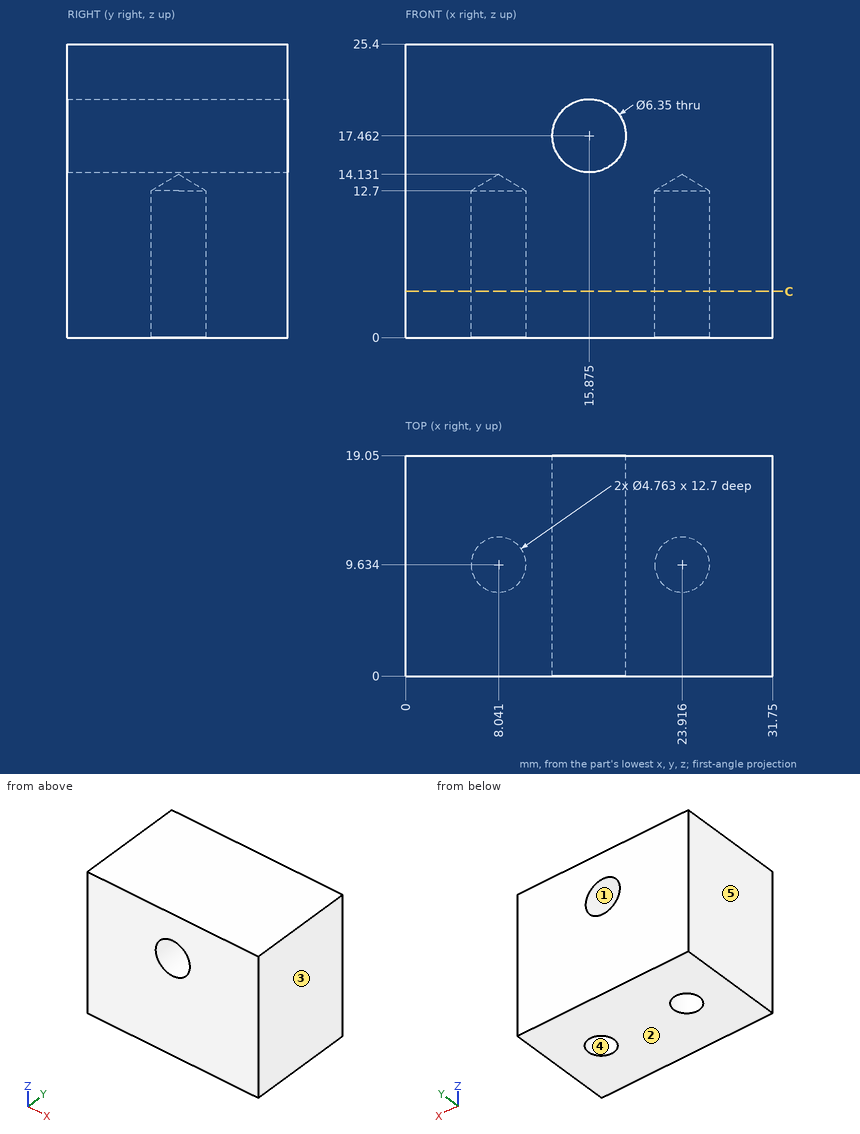
Print and shaded views of the part. All mm, measured from the part's lowest x, y and z. A direction names the side the tool comes from. Round coordinates to 2 decimals unless told otherwise and drop trailing zeros. One line per question, with ' | ' between items.
1. Band-saw the part on C-C, the plane z = 4. Give the number of separate pieces and of enclosed holes in the cut face, and give its area (3 significant figures).
Results are:
separate pieces: 1 | enclosed holes: 2 | area: 569 mm^2
2. Tool access for the marked faces 4 and 5: list every direction of +Z, -Z, +X, -X, +Y, -Y with a clear straight run to the whole face (end or side of a thin tool).
Results are:
face 4: -Z | face 5: +Z, -Z, -X, +Y, -Y
3. Drill centre lines: line 1 along Z through (x, y) = (13.5, 15) (1 decimal); line 2 along X through (y, z) = (13.25, 16.75); line 3 along X through (y, z) = (8, 15.75). Where is each one in solid material? Low to high. Write a range as from..to.
Results are:
line 1: 0..15.4, 19.6..25.4 | line 2: 0..12.78, 18.97..31.75 | line 3: 0..13.2, 18.55..31.75
4. Drop flat-ended pins along their axis: pin 1 Ø4 at (x, z) = (15.88, 17.46) entering from +Y; pin 2 Ø3 at (x, y) = (23.92, 9.63) entering from -Z (1 decimal). Give the stop position or say it passes through.
Results are:
pin 1: through | pin 2: z = 13.2
5. Mould opens along Z. For the marked faces 1, 2 and 3 say: released by +Z, released by -Z, zero draft, split by the parting line, or undercut.
Results are:
face 1: undercut | face 2: released by -Z | face 3: zero draft
